Verification items for the finished model (mm, model axes). Face numbers are marked on the shaded views. A direction names the side the tool comes from. Give positions to 0.01 mm unless a question says otherwise; leave off trailing zeros. Write each loop counter-clockwise with the first axis right and the second up, starting at its lowest first coordinate (ties: lowest second). Pieces come first, ordered by that corner, then holes. Notation, with made-up numbers: (57, 59.25) - (64, 59.25) arc R13 ccw to (64, 76.25) - close; hole circle Ø7 at (-28.5, 63). An arc over 180 degrees is marked (long way). Put each result on its own line as item: value.
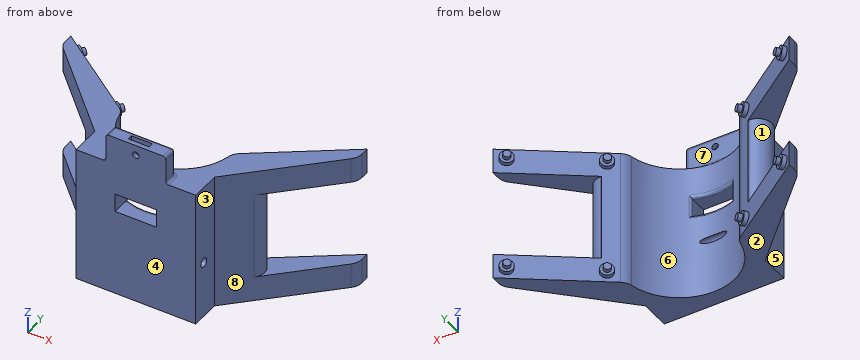
from build123d import *

# Parameters (mm, degrees)
BOSS_EXTRUDE1_DEPTH            = 48
CUT_EXTRUDE2_REACH             = 105.92
SKETCH2_W                      = 61
SKETCH2_H                      = 37.460856798
SKETCH2_R                      = 3.175
CUT_EXTRUDE2_DIRECTION_2_REACH = 105.92
CUT_EXTRUDE3_REACH             = 94.461
SKETCH4_W                      = 29
SKETCH4_H                      = 13
SKETCH5_W                      = 42
SKETCH5_H                      = 10
SKETCH5_W_2                    = 14.7
SKETCH5_H_2                    = 3.5
BOSS_EXTRUDE2_DEPTH            = 20
SKETCH6_R                      = 2.25
CUT_EXTRUDE4_DEPTH             = 11
FILLET1_R                      = 10
FILLET2_R                      = 2
FILLET4_R                      = 2
SKETCH7_R                      = 4.5
SKETCH7_R_2                    = 2.5
BOSS_EXTRUDE3_DEPTH            = 3
SKETCH7_3_R                    = 2.5
BOSS_EXTRUDE4_DEPTH            = 6


with BuildPart() as part:
    # Sketch1 → Boss-Extrude1 (new body, symmetric)
    with BuildSketch(Plane.XY):
        with BuildLine():
            Line((-42, 0), (42, 0))
            Line((42, 0), (42, 21))
            Line((42, 21), (103.920275047, 82.460856798))
            Line((103.920275047, 82.460856798), (103.920275047, 92.460856798))
            Line((103.920275047, 92.460856798), (38.794329483, 46))
            ThreePointArc((38.794329483, 46), (0, 11), (-38.794329483, 46))
            Line((-38.794329483, 46), (-103.920275047, 92.460856798))
            Line((-103.920275047, 92.460856798), (-103.920275047, 82.460856798))
            Line((-103.920275047, 82.460856798), (-42, 21))
            Line((-42, 21), (-42, 0))
        make_face()
    extrude(amount=BOSS_EXTRUDE1_DEPTH, both=True)

    # Sketch2 → Cut-Extrude2 (cut, up to next)
    with BuildSketch(Plane(origin=(0, 0, 0), x_dir=(0, 0, -1), z_dir=(1, 0, 0)), mode=Mode.PRIVATE) as cut_extrude2_sk1:
        with Locations((0, 73.730428399)):
            Rectangle(SKETCH2_W, SKETCH2_H)
    cut_extrude2_tool1 = extrude(cut_extrude2_sk1.sketch, amount=-CUT_EXTRUDE2_REACH, mode=Mode.PRIVATE) & part.part
    add(cut_extrude2_tool1.solids().sort_by_distance((0, 73.730428, 0))[0], mode=Mode.SUBTRACT)
    # Sketch2 → Cut-Extrude2 (cut, up to next)
    with BuildSketch(Plane(origin=(0, 0, 0), x_dir=(0, 0, -1), z_dir=(1, 0, 0)), mode=Mode.PRIVATE) as cut_extrude2_sk2:
        with Locations((8, 9)):
            Circle(SKETCH2_R)
    cut_extrude2_tool2 = extrude(cut_extrude2_sk2.sketch, amount=-CUT_EXTRUDE2_REACH, mode=Mode.PRIVATE) & part.part
    add(cut_extrude2_tool2.solids().sort_by_distance((0, 9, -8))[0], mode=Mode.SUBTRACT)

    # Sketch2 → Cut-Extrude2 direction 2 (cut, up to next)
    with BuildSketch(Plane(origin=(0, 0, 0), x_dir=(0, 0, -1), z_dir=(1, 0, 0)), mode=Mode.PRIVATE) as cut_extrude2_direction_2_sk1:
        with Locations((0, 73.730428399)):
            Rectangle(SKETCH2_W, SKETCH2_H)
    cut_extrude2_direction_2_tool1 = extrude(cut_extrude2_direction_2_sk1.sketch, amount=CUT_EXTRUDE2_DIRECTION_2_REACH, mode=Mode.PRIVATE) & part.part
    add(cut_extrude2_direction_2_tool1.solids().sort_by_distance((0, 73.730428, 0))[0], mode=Mode.SUBTRACT)
    # Sketch2 → Cut-Extrude2 direction 2 (cut, up to next)
    with BuildSketch(Plane(origin=(0, 0, 0), x_dir=(0, 0, -1), z_dir=(1, 0, 0)), mode=Mode.PRIVATE) as cut_extrude2_direction_2_sk2:
        with Locations((8, 9)):
            Circle(SKETCH2_R)
    cut_extrude2_direction_2_tool2 = extrude(cut_extrude2_direction_2_sk2.sketch, amount=CUT_EXTRUDE2_DIRECTION_2_REACH, mode=Mode.PRIVATE) & part.part
    add(cut_extrude2_direction_2_tool2.solids().sort_by_distance((0, 9, -8))[0], mode=Mode.SUBTRACT)

    # Sketch4 → Cut-Extrude3 (cut, up to next)
    with BuildSketch(Plane(origin=(0, 0, 0), x_dir=(1, 0, 0), z_dir=(0, 1, 0)), mode=Mode.PRIVATE) as cut_extrude3_sk1:
        with Locations((0, -19.5)):
            Rectangle(SKETCH4_W, SKETCH4_H)
    cut_extrude3_tool1 = extrude(cut_extrude3_sk1.sketch, amount=CUT_EXTRUDE3_REACH, mode=Mode.PRIVATE) & part.part
    add(cut_extrude3_tool1.solids().sort_by_distance((0, 0, 19.5))[0], mode=Mode.SUBTRACT)

    # Sketch5 → Boss-Extrude2 (add)
    with BuildSketch(Plane.XY.offset(48)):
        with Locations((0, 5)):
            Rectangle(SKETCH5_W, SKETCH5_H)
        with Locations((0, 5)):
            Rectangle(SKETCH5_W_2, SKETCH5_H_2, mode=Mode.SUBTRACT)
    extrude(amount=BOSS_EXTRUDE2_DEPTH)

    # Sketch6 → Cut-Extrude4 (cut, through all)
    with BuildSketch(Plane(origin=(0, 10, 0), x_dir=(1, 0, 0), z_dir=(0, 1, 0))):
        with Locations((0, -60.885403607)):
            Circle(SKETCH6_R)
    extrude(amount=-CUT_EXTRUDE4_DEPTH, mode=Mode.SUBTRACT)

    # Fillet1
    fillet1_edges = [part.edges().sort_by_distance(p)[0] for p in [
        (-103.920275047, 82.460856798, -39.25),
        (-38.794329483, 46, 0),
        (38.794329483, 46, 0),
        (103.920275047, 82.460856798, -39.25),
        (103.920275047, 82.460856798, 39.25),
        (-103.920275047, 82.460856798, 39.25),
        (76.254149084, 55, 0),
        (-76.254149084, 55, 0),
    ]]
    fillet(fillet1_edges, radius=FILLET1_R)

    # Fillet2
    fillet2_edges = [part.edges().sort_by_distance(p)[0] for p in [
        (0, 11, 26),
        (14.5, 13.795718485, 19.5),
        (0, 11, 13),
        (-14.5, 13.795718485, 19.5),
    ]]
    fillet(fillet2_edges, radius=FILLET2_R)

    # Fillet4
    fillet4_edges = [part.edges().sort_by_distance(p)[0] for p in [
        (21, 5, 68),
        (0, 10, 68),
        (-21, 5, 68),
        (21, 5, 48),
        (0, 10, 48),
        (21, 10, 58),
        (-21, 5, 48),
        (-21, 10, 58),
    ]]
    fillet(fillet4_edges, radius=FILLET4_R)

    # Sketch7 → Boss-Extrude3 (add)
    with BuildSketch(Plane(origin=(-8.663321552, 12.143706482, 0), x_dir=(0.81407432, 0.58076071, 0), z_dir=(-0.58076071, 0.81407432, 0))):
        with Locations((130.296460035, -40.5)):
            Circle(SKETCH7_R)
        with Locations((130.296460035, -40.5)):
            Circle(SKETCH7_R_2, mode=Mode.SUBTRACT)
        with Locations((70.606460035, -40.5)):
            Circle(SKETCH7_R)
        with Locations((70.606460035, -40.5)):
            Circle(SKETCH7_R_2, mode=Mode.SUBTRACT)
        with Locations((130.296460035, 40.78)):
            Circle(SKETCH7_R)
        with Locations((130.296460035, 40.78)):
            Circle(SKETCH7_R_2, mode=Mode.SUBTRACT)
        with Locations((70.606460035, 40.78)):
            Circle(SKETCH7_R)
        with Locations((70.606460035, 40.78)):
            Circle(SKETCH7_R_2, mode=Mode.SUBTRACT)
    boss_extrude3 = extrude(amount=BOSS_EXTRUDE3_DEPTH)

    # Sketch7_3 → Boss-Extrude4 (add)
    with BuildSketch(Plane(origin=(-8.663321552, 12.143706482, 0), x_dir=(0.81407432, 0.58076071, 0), z_dir=(-0.58076071, 0.81407432, 0))):
        with Locations((70.606460035, -40.5)):
            Circle(SKETCH7_3_R)
        with Locations((70.606460035, 40.78)):
            Circle(SKETCH7_3_R)
        with Locations((130.296460035, 40.78)):
            Circle(SKETCH7_3_R)
        with Locations((130.296460035, -40.5)):
            Circle(SKETCH7_3_R)
    boss_extrude4 = extrude(amount=BOSS_EXTRUDE4_DEPTH)

    # Mirror1: Boss-Extrude3, Boss-Extrude4 across plane
    add(boss_extrude3.mirror(Plane(origin=(0, 0, 0), x_dir=(0, 0, 1), z_dir=(1, 0, 0))))
    add(boss_extrude4.mirror(Plane(origin=(0, 0, 0), x_dir=(0, 0, 1), z_dir=(1, 0, 0))))


solid = part.part
Q1. Section check C-C, the plane y = 18.5. Record the cut outline in (x, z), plus the area to 3 significant figures.
Answers follow:
outline: (-42, -48) - (-22.99, -48) - (-22.99, 48) - (-42, 48) - close; (22.99, -48) - (42, -48) - (42, 48) - (22.99, 48) - close
area: 3,650 mm2
Q2. Set-up check for the marked faces 1, 2, 3, 4 and 5: record each of +Z, -Z, +X, -X, +Y, -Y from which the full face is reachable in a straight line by a thin tool's end or side.
Answers follow:
face 1: -X
face 2: -Z, +X, -X, +Y, -Y
face 3: +Z, -Z, +X, -Y
face 4: +Z, -Z, +X, -X, -Y
face 5: +Z, -Z, -X, -Y
Q3. Section check A-A, the plane y = 70.5. Record the cut outline in (x, z), plus the area to 3 significant figures.
Answers follow:
outline: (-91.87, -48) - (-73.14, -48) - (-73.14, -30.5) - (-91.87, -30.5) - close; (-91.87, 30.5) - (-73.14, 30.5) - (-73.14, 48) - (-91.87, 48) - close; (73.14, -48) - (91.87, -48) - (91.87, -30.5) - (73.14, -30.5) - close; (73.14, 30.5) - (91.87, 30.5) - (91.87, 48) - (73.14, 48) - close
area: 1,310 mm2
Q4. Scan lines: line 1 along Z through (x, y) = (0, 1.95); line 2 along Z through (x, y) = (61, 54); line 3 along X through (y, z) = (34, 43). Record each from-to range of solid material in increasing order.
Answers follow:
line 1: z = -48 to 13, 26 to 58.64, 63.14 to 68
line 2: z = -48 to -30.5, 30.5 to 48
line 3: x = -55.1 to -35.57, 35.57 to 55.1
Q5. Section check D-D, the plane x = -34. Record the cut outline in (y, z) (3 decimals), plus the area to 3 significant figures.
Answers follow:
outline: (0, -48) - (30.895, -48) - (30.895, 48) - (0, 48) - close; hole circle Ø6.35 at (9, -8)
area: 2,930 mm2
Q6. Go/stop test with flat-tipped pins: pin 1 Ø10 at (y, z) = (7, 22) entering from -X; pin 2 Ø13 at (x, z) = (7.5, 57.5) entering from +Y; pin 3 Ø3.5 at (x, z) = (0, 60.89) entering from -Y; pin 4 Ø8 at (y, z) = (53.5, 41) entering from -X. Record where each tip stops, or that it passes through.
Answers follow:
pin 1: stops at x = -42
pin 2: stops at y = 10
pin 3: passes through
pin 4: stops at x = -78.77
Q7. Section check B-B, the plane z = -8. Record the cut outline in (x, y) (1 decimal), plus the area to 3 significant figures.
Answers follow:
outline: (-59, 37.9) - (-42, 21) - (-42, 12.2) - (-9.5, 12.2) arc R39 cw to (-38.2, 42.3) arc R10 ccw to (-42.2, 48.4) - (-51.4, 55) - (-52, 55) arc R10 ccw to start; (-42, 0) - (42, 0) - (42, 5.8) - (-42, 5.8) - close; (9.5, 12.2) - (42, 12.2) - (42, 21) - (59, 37.9) arc R10 ccw to (52, 55) - (51.4, 55) - (42.2, 48.4) arc R10 ccw to (38.2, 42.3) arc R39 cw to start
area: 2,120 mm2
Q8. Release check for a two-part mould opening along X. For the marked faces 6, 7 and 8 record: released by +X, released by -X, zero draft, split by the parting line, or undercut.
Answers follow:
face 6: undercut
face 7: zero draft
face 8: released by +X
